The listing builds one solid part. Answer for the finished solid, in the listing's coordinates (mm). Give positions to 0.01 mm unless a question says otherwise; leave off trailing zeros. Order: outer loops, then holes, each group sorted by start corner. A loop starts at its lowest first (then second) coordinate and runs counter-clockwise, first axis right, second up. Notation, with made-up numbers: (-24.75, -34) - (26.25, -34) arc R13 cw to (26.25, -30) - close; hole circle Ø10 at (32.5, 38.25). An arc over 180 degrees is marked (long way). Answer in a Markdown table with one row per item.
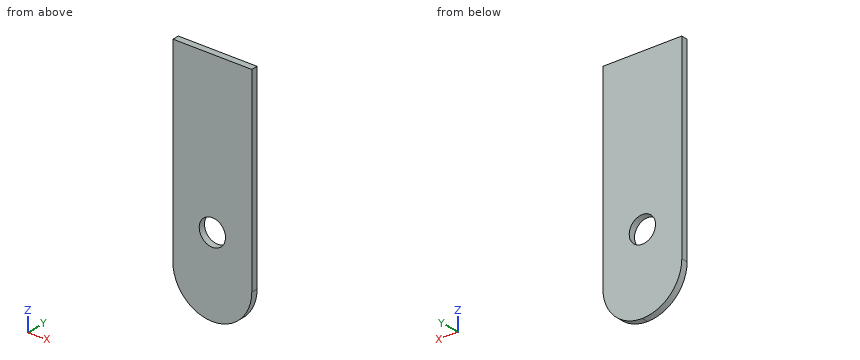
from build123d import *

# Parameters (mm, degrees)
SKETCH1_W           = 76.2
SKETCH1_H           = 228.6
SKETCH1_R           = 12.7
BOSS_EXTRUDE1_DEPTH = 6.35
FILLET1_R           = 38.1


with BuildPart() as part:
    # Sketch1 → Boss-Extrude1 (new body)
    with BuildSketch(Plane(origin=(0, 0, 0), x_dir=(-1, 0, 0), z_dir=(0, 1, 0))):
        Rectangle(SKETCH1_W, SKETCH1_H)
        with Locations(Location((0, -38.1, 0), (0, 0, 90))):
            Circle(SKETCH1_R, mode=Mode.SUBTRACT)
    extrude(amount=BOSS_EXTRUDE1_DEPTH)

    # Fillet1
    fillet1_edges = [part.edges().sort_by_distance(p)[0] for p in [
        (-38.1, 3.175, -114.3),
        (38.1, 3.175, -114.3),
    ]]
    fillet(fillet1_edges, radius=FILLET1_R - 0.0001)  # a hair under: the kernel refuses the full size


solid = part.part
Item 1: Find section C-C on x = -9. Write down the section's boundary in (y, z).
Answer block:
| item | result |
|---|---|
| outline | (0, -113.22) - (6.35, -113.22) - (6.35, -47.06) - (0, -47.06) - close; (0, -29.14) - (6.35, -29.14) - (6.35, 114.3) - (0, 114.3) - close |
Item 2: Find section B-B on z = -38.1. Write down the section's boundary in (x, y).
Answer block:
| item | result |
|---|---|
| outline | (-38.1, 0) - (-12.7, 0) - (-12.7, 6.35) - (-38.1, 6.35) - close; (12.7, 0) - (38.1, 0) - (38.1, 6.35) - (12.7, 6.35) - close |
Item 3: This flat-tipped pin is pushed along its axis until it touches: P1, Ø3, axis at y = 2, z = -89, coming from the +X side. Where does it stop, or does it pass through?
Answer block:
| item | result |
|---|---|
| P1 | x = 36.39 |
Item 4: Consider line 1 (X direction, y = 4.5, z = -38.1); line 2 (X direction, y = 6, z = -29.5); line 3 (Z direction, x = -8, y = 3). Determine where each line is inside the solid, lowest interval first.
Answer block:
| item | result |
|---|---|
| line 1 | -38.1 to -12.7, 12.7 to 38.1 |
| line 2 | -38.1 to -9.35, 9.35 to 38.1 |
| line 3 | -113.45 to -47.96, -28.24 to 114.3 |
Item 5: Find section D-D on x = 18. Write down the section's boundary in (y, z), then the cut area to 3 significant figures.
Answer block:
| item | result |
|---|---|
| outline | (0, -109.78) - (6.35, -109.78) - (6.35, 114.3) - (0, 114.3) - close |
| area | 1,420 mm² |
